For this review, use the dimensioned drawing (mm, ordinates from the lowest corner) and the shaded views. A direction names the side the tool comes from. Coordinates: 2 decimals unless noted, no trailing zeros. Loops run counter-clockwise (first coordinate to the right, second up) from the corner with the lowest first, then second, coordinate; pieces in that order, holes last. Notation, with made-up numbers: M 3,87.5 L 38,87.5 A24 cw 38,122.5 Z; hole C -19,-12.5 d5. An arc over 180 degrees is marked long. One line per item, written item: value.
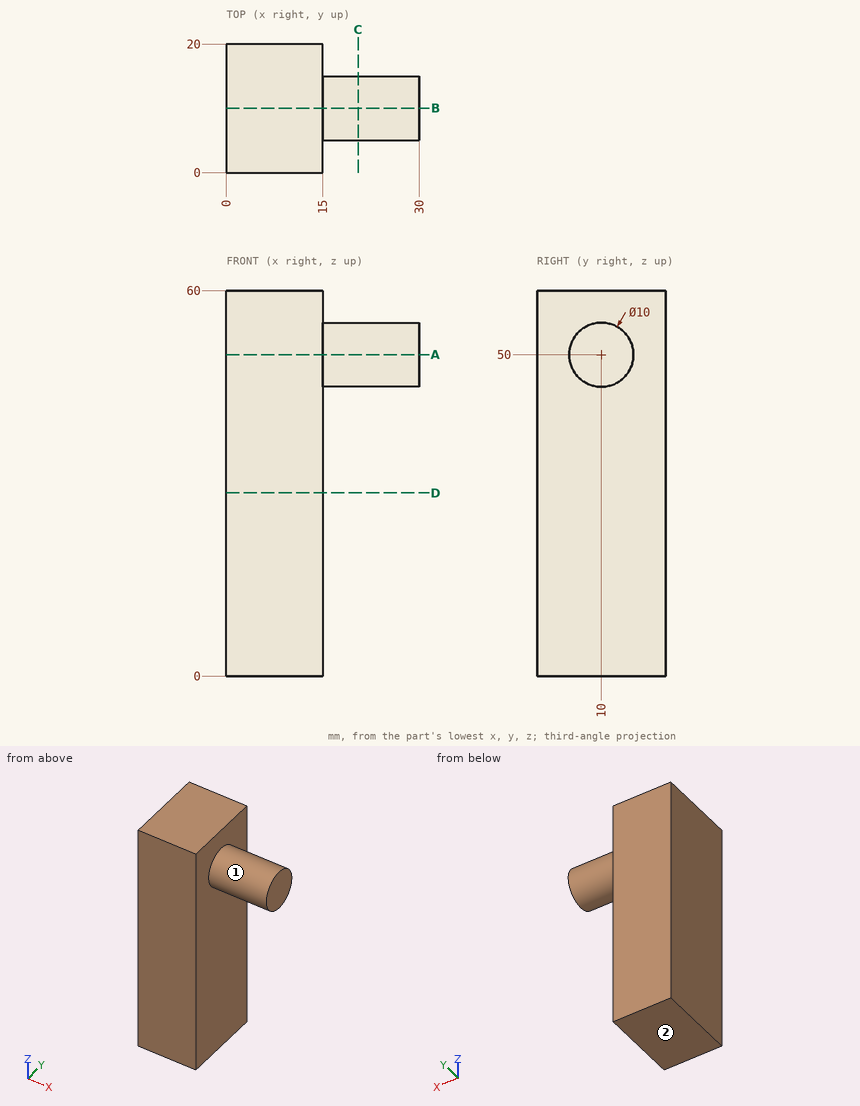
(1) Add section A-A on z = 50. State the section outline as (x, y) points, then the cut area to 3 significant figures.
Checks:
outline: M 0,0 L 15,0 L 15,5 L 30,5 L 30,15 L 15,15 L 15,20 L 0,20 Z
area: 450 mm^2
(2) Insertion check: pin 1 Ø2 at (x, y) = (22, 5.5) entering from -Z; pin 2 Ø6 at (y, z) = (12, 40.5) entering from +X; pin 3 Ø6 at (x, y) = (26.5, 7.5) entering from +Z. Each pin has a flat end and moves straight along its axis. Give the tip position at first contact, or say it passes through.
Checks:
pin 1: z = 46.43
pin 2: x = 15
pin 3: z = 55
(3) To check wall thickness, follow L1, parallel to X at y = 8, z = 39; L2, parallel to Z at x = 20.5, y = 11.5; L3, parallel to Z at x = 19, y = 6.5. State the ranges of each line that lie inside material, in increasing order. Write a range as [from, to].
Checks:
L1: [0, 15]
L2: [45.23, 54.77]
L3: [46.43, 53.57]
(4) Add section D-D on z = 28.5. State the section outline as (x, y) points, then the cut area to 3 significant figures.
Checks:
outline: M 0,0 L 15,0 L 15,20 L 0,20 Z
area: 300 mm^2
(5) Add section B-B on y = 10. State the section outline as (x, z) points, then the cut area to 3 significant figures.
Checks:
outline: M 0,0 L 15,0 L 15,45 L 30,45 L 30,55 L 15,55 L 15,60 L 0,60 Z
area: 1,050 mm^2
(6) Add section C-C on x = 20.5. State the section outline as (y, z) points.
Checks:
outline: C 10,50 d10
(7) Tool access review of the marked faces 1 and 2: name each direction out of +Z, -Z, +X, -X, +Y, -Y from which nothing blocks a thin tool from reaching the whole face with its end or side.
Checks:
face 1: +X
face 2: -Z, +X, -X, +Y, -Y
